Check sheet for the modelled part. Datum: model origin and axes. Units: mm. Round coordinates to 2 decimals unless told otherwise and drop trailing zeros. Write each loop counter-clockwise with the first axis right and the second up, starting at its lowest first coordinate (ties: lowest second). Pieces come first, ordered by that corner, then holes. Notation, with made-up numbers: (30.5, 82) -> (35.5, 82) arc R33 ccw to (35.5, 117) -> close; hole circle Ø9 at (15, 66). An arc over 180 degrees is marked (long way). One line per item, written item: value.
from build123d import *

# Parameters (mm, degrees)
BOSS_EXTRU_1_DEPTH = 24


with BuildPart() as part:
    # Esquisse3 → Boss.-Extru.1 (new body)
    with BuildSketch(Plane(origin=(0, 0, 0), x_dir=(1, 0, 0), z_dir=(0, 1, 0))):
        Polygon((3, 0), (1.5, 2.598076211), (-1.5, 2.598076211), (-3, 0), (-1.5, -2.598076211), (1.5, -2.598076211), align=None)
    extrude(amount=BOSS_EXTRU_1_DEPTH)


solid = part.part
Item 1: Material ranges on line 1 along X through (y, z) = (22.75, -2.2); line 2 along Z through (x, y) = (1.9, 18.5); line 3 along Z through (x, y) = (2.1, 19.5), recorded low to high.
Result set:
line 1: -1.73 to 1.73
line 2: -1.91 to 1.91
line 3: -1.56 to 1.56
Item 2: Sectioned sample at A-A (y = 20.25). Enter the section's corners in (x, z), then the cut area to 3 significant figures.
Result set:
outline: (-3, 0) -> (-1.5, -2.6) -> (1.5, -2.6) -> (3, 0) -> (1.5, 2.6) -> (-1.5, 2.6) -> close
area: 23.4 mm^2
Item 3: Sectioned sample at C-C (x = -1.9). Enter the section's corners in (y, z), then the cut area to 3 significant figures.
Result set:
outline: (0, -1.91) -> (24, -1.91) -> (24, 1.91) -> (0, 1.91) -> close
area: 91.5 mm^2
Item 4: Sectioned sample at B-B (z = 1.4). Enter the section's corners in (x, y), then the cut area to 3 significant figures.
Result set:
outline: (-2.19, 0) -> (2.19, 0) -> (2.19, 24) -> (-2.19, 24) -> close
area: 105 mm^2
